For this review, take the finished solid that the model builds, in its own axes (mm). Face numbers are marked on the shaded views. A direction names the side the tool comes from. Coordinates: 2 decimals unless noted, no trailing zeros. Write each loop counter-clockwise with the first axis right and the second up, starting at its lowest first coordinate (ties: lowest second). Pieces come first, ordered by that corner, then holes.
```python
from build123d import *

# Parameters (mm, degrees)
CROQUIS1_R              = 5
CROQUIS1_R_2            = 3.75
SALIENTE_EXTRUIR3_DEPTH = 10
REDONDEO3_R             = 5
CROQUIS3_R              = 2
SALIENTE_EXTRUIR4_DEPTH = 10


with BuildPart() as part:
    # Croquis1 → Saliente-Extruir3 (new body)
    # profile 1 of 5: a face of its own
    with BuildSketch(Plane(origin=(0, 0, 0), x_dir=(1, 0, 0), z_dir=(0, 1, 0))):
        with BuildLine():
            ThreePointArc((6.179553234, 26.796699831), (0, 27.5), (-6.179553234, 26.796699831))
            Line((-6.179553234, 26.796699831), (-26.296399408, -8.046699831))
            ThreePointArc((-26.296399408, -8.046699831), (-23.815698604, -13.75), (-20.116846174, -18.75))
            Line((-20.116846174, -18.75), (20.116846174, -18.75))
            ThreePointArc((20.116846174, -18.75), (23.815698604, -13.75), (26.296399408, -8.046699831))
            Line((26.296399408, -8.046699831), (6.179553234, 26.796699831))
        make_face()
        with Locations(Location((-15.155444566, -8.75, 0), (0, 0, 270))):
            Circle(CROQUIS1_R, mode=Mode.SUBTRACT)
        with Locations(Location((15.155444566, -8.75, 0), (0, 0, 270))):
            Circle(CROQUIS1_R, mode=Mode.SUBTRACT)
        with BuildLine():
            ThreePointArc((0, 7.5), (2.053290038, 7.406507449), (3.995190528, 8.080127019))
            ThreePointArc((3.995190528, 8.080127019), (1.58501754, 10.938896501), (-1.666208496, 12.785792829))
            ThreePointArc((-1.666208496, 12.785792829), (-4.714207171, 19.166208496), (1.666208496, 22.214207171))
            ThreePointArc((1.666208496, 22.214207171), (7.977102724, 18.629231149), (12.655444566, 13.080127019))
            Line((12.655444566, 13.080127019), (17.655444566, 4.419872981))
            Line((17.655444566, 4.419872981), (8.995190528, -0.580127019))
            ThreePointArc((8.995190528, -0.580127019), (7.440868623, -1.92505239), (6.495190528, -3.75))
            ThreePointArc((6.495190528, -3.75), (0, -6.171567416), (-6.495190528, -3.75))
            ThreePointArc((-6.495190528, -3.75), (-5.344734164, 3.085783708), (0, 7.5))
        make_face(mode=Mode.SUBTRACT)
    # profile 2 of 5: a face of its own
    with BuildSketch(Plane(origin=(0, 0, 0), x_dir=(1, 0, 0), z_dir=(0, 1, 0))):
        with BuildLine():
            ThreePointArc((0, 7.5), (5.344734164, 3.085783708), (6.495190528, -3.75))
            ThreePointArc((6.495190528, -3.75), (0, -6.171567416), (-6.495190528, -3.75))
            ThreePointArc((-6.495190528, -3.75), (-5.344734164, 3.085783708), (0, 7.5))
        make_face()
        with Locations(Location((0, 0, 0), (0, 0, 270))):
            Circle(CROQUIS1_R_2, mode=Mode.SUBTRACT)
    # profile 3 of 5: a face of its own
    with BuildSketch(Plane(origin=(0, 0, 0), x_dir=(1, 0, 0), z_dir=(0, 1, 0))):
        with BuildLine():
            ThreePointArc((8.995190528, -0.580127019), (7.440868623, -1.92505239), (6.495190528, -3.75))
            ThreePointArc((6.495190528, -3.75), (5.344734164, 3.085783708), (0, 7.5))
            ThreePointArc((0, 7.5), (2.053290038, 7.406507449), (3.995190528, 8.080127019))
            Line((3.995190528, 8.080127019), (8.995190528, -0.580127019))
        make_face()
    # profile 4 of 5: a face of its own
    with BuildSketch(Plane(origin=(0, 0, 0), x_dir=(1, 0, 0), z_dir=(0, 1, 0))):
        Polygon((17.655444566, 4.419872981), (8.995190528, -0.580127019), (3.995190528, 8.080127019), (12.655444566, 13.080127019), align=None)
    # profile 5 of 5: a face of its own
    with BuildSketch(Plane(origin=(0, 0, 0), x_dir=(1, 0, 0), z_dir=(0, 1, 0))):
        with BuildLine():
            ThreePointArc((-1.666208496, 12.785792829), (1.58501754, 10.938896501), (3.995190528, 8.080127019))
            Line((3.995190528, 8.080127019), (12.655444566, 13.080127019))
            ThreePointArc((12.655444566, 13.080127019), (7.977102724, 18.629231149), (1.666208496, 22.214207171))
            ThreePointArc((1.666208496, 22.214207171), (4.082342617, 20.386949733), (5, 17.5))
            ThreePointArc((5, 17.5), (2.886949733, 13.417657383), (-1.666208496, 12.785792829))
        make_face()
    extrude(amount=SALIENTE_EXTRUIR3_DEPTH)

    # Redondeo3
    redondeo3_edges = [part.edges().sort_by_distance(p)[0] for p in [
        (-20.116846174, 5, 18.75),
        (-26.296399408, 5, 8.046699831),
        (-6.179553234, 5, -26.796699831),
        (6.179553234, 5, -26.796699831),
        (26.296399408, 5, 8.046699831),
        (20.116846174, 5, 18.75),
    ]]
    fillet(redondeo3_edges, radius=REDONDEO3_R)

    # Croquis3 → Saliente-Extruir4 (add)
    with BuildSketch(Plane.XZ):
        with Locations(Location((23.805967574, 8.75, 0), (0, 0, 3.846633593))):
            Circle(CROQUIS3_R)
        with Locations(Location((-4.325261504, -24.99157268, 0), (0, 0, 243.846633832))):
            Circle(CROQUIS3_R)
        with Locations(Location((-19.48070607, 16.24157268, 0), (0, 0, 123.846633623))):
            Circle(CROQUIS3_R)
    extrude(amount=SALIENTE_EXTRUIR4_DEPTH)


solid = part.part
```
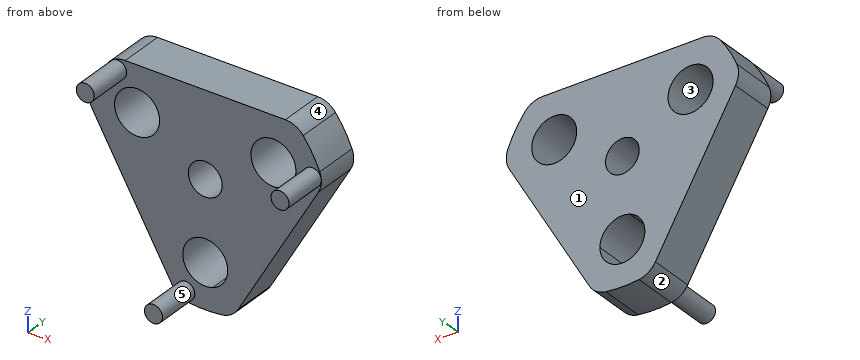
1) Clearance check with flat-ended pins moving along their axes: P1, Ø8, axis at y = -1, z = -4, coming from the -X side; P2, Ø2, axis at x = 2, y = 4, coming from the -Z side; P3, Ø3, axis at y = 7.5, z = -2, coming from the -X side. State where each tip first meets the part, or that it passes through.
2) Tool access review of the marked faces 4 and 5: name each direction out of +Z, -Z, +X, -X, +Y, -Y from which nothing blocks a thin tool from reaching the whole face with its end or side.
3) For L1, parallel to X at y = 4.5, z = 8.75; L2, parallel to X at y = 0.5, z = 13; L3, parallel to Z at x = -2.5, y = 5.25, list the stretches that pass through material, from the lowest coordinate up.
4) Consider section B-B (z = 0). Give the boundary of the cut face in (x, y).
5) Consider section D-D (y = 8.75). Give the boundary of the cut face in (x, z), then the cut area to 3 significant figures.
6) The part is to be moulded in two halves that separate along X. For the marked faces 1, 2 and 3, say which applies: pulls with the +X half, pulls with the -X half, needs draft (parallel to the pull), parting line crosses it, or undercut.
7) Consider section A-A (x = 0). Give the boundary of the cut face in (y, z).
8) Consider section C-C (x = 14). Give the boundary of the cut face in (y, z), then the cut area to 3 significant figures.
Results:
1. P1: stops at x = -21.58
1. P2: stops at z = -27.48
1. P3: stops at x = -21.36
2. face 4: +Z, +X, +Y, -Y
2. face 5: -Y
3. L1: x = -25.81 to -20.16, -10.16 to 10.16, 20.16 to 25.81
3. L2: x = -24.23 to -17.79, -12.52 to 12.52, 17.79 to 24.23
3. L3: z = -27.39 to -21.83, -13.17 to -2.8, 2.8 to 18.75
4. outline: (-21.65, 0) - (-3.75, 0) - (-3.75, 10) - (-21.65, 10) - close; (3.75, 0) - (21.65, 0) - (21.65, 10) - (3.75, 10) - close
5. outline: (-25.44, 10.45) arc R5 ccw to (-25.14, 6.05) - (-7.33, -24.8) arc R5 ccw to (-3.67, -27.25) arc R27.5 ccw to (3.67, -27.25) arc R5 ccw to (7.33, -24.8) - (25.14, 6.05) arc R5 ccw to (25.44, 10.45) arc R27.5 ccw to (21.77, 16.81) arc R5 ccw to (17.81, 18.75) - (-17.81, 18.75) arc R5 ccw to (-21.77, 16.81) arc R27.5 ccw to start; hole circle Ø10 at (-15.16, 8.75); hole circle Ø10 at (0, -17.5); hole circle Ø7.5 at (0, 0); hole circle Ø10 at (15.16, 8.75)
5. area: 1,360 mm2
6. face 1: needs draft
6. face 2: pulls with the -X half
6. face 3: undercut
7. outline: (0, -27.5) - (10, -27.5) - (10, -22.5) - (0, -22.5) - close; (0, -12.5) - (10, -12.5) - (10, -3.75) - (0, -3.75) - close; (0, 3.75) - (10, 3.75) - (10, 18.75) - (0, 18.75) - close
8. outline: (0, -13.25) - (10, -13.25) - (10, 3.89) - (0, 3.89) - close; (0, 13.61) - (10, 13.61) - (10, 18.75) - (0, 18.75) - close
8. area: 223 mm2
